For this review, take the finished solid that the model builds, in its own axes (mm). Face numbers are marked on the shaded views. A direction names the side the tool comes from. Give positions to 0.01 mm unless a question says otherwise; leave off trailing zeros. Write each loop counter-clockwise with the first axis right and the second up, starting at its lowest first coordinate (ties: lowest second). Pieces come first, ordered by that corner, then holes. Notation, with made-up numbers: M -16.5,-37.75 L 36.5,-37.75 A26 ccw 36.5,-15.75 Z; hole C 30,9.25 d7. An arc over 180 degrees is marked long. One line per item, written item: value. Start each with the question number.
Item 1: Tool access review of the marked faces 4 and 5: name each direction out of +Z, -Z, +X, -X, +Y, -Y from which nothing blocks a thin tool from reaching the whole face with its end or side.
Item 2: Consider section C-C, the plane z = 35.5. Write out the cut boundary in (x, y).
Item 3: Clearance check with flat-ended pins moving along their axes: pin 1 Ø0.6 at (y, z) = (3.5, 15.5) entering from +X; pin 2 Ø2 at (x, y) = (1, 2.5) entering from -Z; pin 3 Ø1.9 at (y, z) = (-3.5, 4.5) entering from -X; pin 4 Ø0.9 at (x, z) = (0, 2.75) entering from +Y. State where each tip first meets the part, or that it passes through.
Item 4: Consider section B-B, the plane z = 4.5. Write out the cut boundary in (x, y).
Item 5: To check wall thickness, follow probe 1 along X at (y, z) = (-4.95, 2.75); probe 2 along Z at (x, y) = (0, -4.35); probe 3 along Y at (x, z) = (2.25, 35.5). State the ranges of each line that lie inside material, in increasing order.
Item 6: Mouldability with a two-part tool opening along Y and no side actions: class the marked faces 1, 2 and 3 as released by +Y, released by -Y, zero draft, split by the parting line, or undercut.
Item 7: Consider section A-A, the plane x = 0. Write out the cut boundary in (y, z).
Item 8: Consider section D-D, the plane y = -4.25. Write out the cut boundary in (x, z), and give its area (3 significant figures).
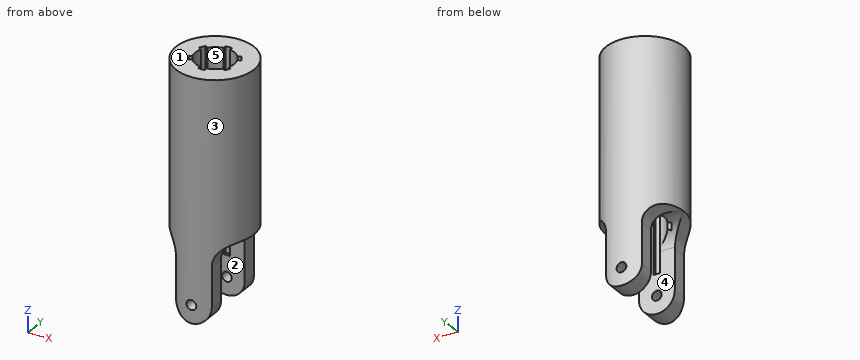
```python
from build123d import *

# Parameters (mm, degrees)
SKETCH_1_R          = 6
SKETCH_1_R_2        = 2.5
EXTRUDE_1_DEPTH     = 37
SKETCH_2_OUTSIDE_W  = 22.142
SKETCH_2_OUTSIDE_H  = 47.142
SKETCH_2_OUTSIDE_R  = 0.75
CUT_EXTRUDE_1_DEPTH = 9.5
CUT_EXTRUDE_2_DEPTH = 9.5
CUT_EXTRUDE_3_DEPTH = 31


with BuildPart() as part:
    # 草图1 → 凸台-拉伸1 (new body)
    with BuildSketch(Plane.XY):
        Circle(SKETCH_1_R)
        Circle(SKETCH_1_R_2, mode=Mode.SUBTRACT)
    extrude(amount=EXTRUDE_1_DEPTH)

    # 草图2 outside → 切除-拉伸1 (cut, symmetric)
    with BuildSketch(Plane(origin=(0, 0, 0), x_dir=(1, 0, 0), z_dir=(0, 1, 0))):
        with Locations((0, -18.5)):
            Rectangle(SKETCH_2_OUTSIDE_W, SKETCH_2_OUTSIDE_H)
        with BuildLine():
            Line((-2.75, -2.75), (-2.75, -9))
            ThreePointArc((-2.75, -9), (-3.701902961, -11.298097039), (-6, -12.25))
            Line((-6, -12.25), (-6, -37))
            Line((-6, -37), (6, -37))
            Line((6, -37), (6, -12.25))
            ThreePointArc((6, -12.25), (3.701902961, -11.298097039), (2.75, -9))
            Line((2.75, -9), (2.75, -2.75))
            ThreePointArc((2.75, -2.75), (0, 0), (-2.75, -2.75))
        make_face(mode=Mode.SUBTRACT)
        with Locations((0, -2.75)):
            Circle(SKETCH_2_OUTSIDE_R)
    extrude(amount=CUT_EXTRUDE_1_DEPTH, both=True, mode=Mode.SUBTRACT)

    # 草图3 → 切除-拉伸2 (cut, symmetric)
    with BuildSketch(Plane(origin=(0, 0, 0), x_dir=(0, 0, -1), z_dir=(1, 0, 0))):
        with BuildLine():
            Line((-9.250000001, 3), (0.966464558, 3))
            Line((0.966464558, 3), (0.966464558, -3))
            Line((0.966464558, -3), (-9.250000001, -3))
            ThreePointArc((-9.250000001, -3), (-12.250000001, 0), (-9.250000001, 3))
        make_face()
    extrude(amount=CUT_EXTRUDE_2_DEPTH, both=True, mode=Mode.SUBTRACT)

    # 草图4 → 切除-拉伸3 (cut)
    with BuildSketch(Plane.XY.offset(37)):
        with BuildLine():
            Line((-0.5, 3.464101615), (-0.5, 2.958039892))
            ThreePointArc((-0.5, 2.958039892), (-1.5, 2.598076211), (-2.311737691, 1.912032648))
            Line((-2.311737691, 1.912032648), (-2.75, 2.165063509))
            ThreePointArc((-2.75, 2.165063509), (-3.031088913, 1.75), (-3.25, 1.299038106))
            Line((-3.25, 1.299038106), (-2.811737691, 1.046007244))
            ThreePointArc((-2.811737691, 1.046007244), (-3, 0), (-2.811737691, -1.046007244))
            Line((-2.811737691, -1.046007244), (-3.25, -1.299038106))
            ThreePointArc((-3.25, -1.299038106), (-3.031088913, -1.75), (-2.75, -2.165063509))
            Line((-2.75, -2.165063509), (-2.311737691, -1.912032648))
            ThreePointArc((-2.311737691, -1.912032648), (-1.5, -2.598076211), (-0.5, -2.958039892))
            Line((-0.5, -2.958039892), (-0.5, -3.464101615))
            ThreePointArc((-0.5, -3.464101615), (0, -3.5), (0.5, -3.464101615))
            Line((0.5, -3.464101615), (0.5, -2.958039892))
            ThreePointArc((0.5, -2.958039892), (1.5, -2.598076211), (2.311737691, -1.912032648))
            Line((2.311737691, -1.912032648), (2.75, -2.165063509))
            ThreePointArc((2.75, -2.165063509), (3.031088913, -1.75), (3.25, -1.299038106))
            Line((3.25, -1.299038106), (2.811737691, -1.046007244))
            ThreePointArc((2.811737691, -1.046007244), (3, 0), (2.811737691, 1.046007244))
            Line((2.811737691, 1.046007244), (3.25, 1.299038106))
            ThreePointArc((3.25, 1.299038106), (3.031088913, 1.75), (2.75, 2.165063509))
            Line((2.75, 2.165063509), (2.311737691, 1.912032648))
            ThreePointArc((2.311737691, 1.912032648), (1.5, 2.598076211), (0.5, 2.958039892))
            Line((0.5, 2.958039892), (0.5, 3.464101615))
            ThreePointArc((0.5, 3.464101615), (0, 3.5), (-0.5, 3.464101615))
        make_face()
    extrude(amount=-CUT_EXTRUDE_3_DEPTH, mode=Mode.SUBTRACT)


solid = part.part
```
Model answer:
1. face 4: -Z, +X, -X
1. face 5: +Z, -Z
2. outline: C 0,0 d12; hole M -3.25,-1.3 A3.5 ccw -2.75,-2.17 L -2.31,-1.91 A3 ccw -0.5,-2.96 L -0.5,-3.46 A3.5 ccw 0.5,-3.46 L 0.5,-2.96 A3 ccw 2.31,-1.91 L 2.75,-2.17 A3.5 ccw 3.25,-1.3 L 2.81,-1.05 A3 ccw 2.81,1.05 L 3.25,1.3 A3.5 ccw 2.75,2.17 L 2.31,1.91 A3 ccw 0.5,2.96 L 0.5,3.46 A3.5 ccw -0.5,3.46 L -0.5,2.96 A3 ccw -2.31,1.91 L -2.75,2.17 A3.5 ccw -3.25,1.3 L -2.81,1.05 A3 ccw -2.81,-1.05 Z
3. pin 1: stops at x = 5.08
3. pin 2: stops at z = 0
3. pin 3: stops at x = -2.75
3. pin 4: passes through
4. outline: M -2.75,-5.33 A6 ccw 2.75,-5.33 L 2.75,-3 L -2.75,-3 Z; M -2.75,3 L 2.75,3 L 2.75,5.33 A6 ccw -2.75,5.33 Z
5. probe 1: x = -2.75 to -0.75, 0.75 to 2.75
5. probe 2: z = 0 to 2, 3.5 to 37
5. probe 3: y = -5.56 to -1.98, 1.98 to 5.56
6. face 1: zero draft
6. face 2: undercut
6. face 3: split by the parting line
7. outline: M -6,0 L -3,0 L -3,2 L -6,2 Z; M -6,3.5 L -3,3.5 L -3,6 L -3.5,6 L -3.5,37 L -6,37 Z; M 3,0 L 6,0 L 6,2 L 3,2 Z; M 3,3.5 L 6,3.5 L 6,37 L 3.5,37 L 3.5,6 L 3,6 Z
8. outline: M -4.24,11.73 A3.25 cw -2.75,9 L -2.75,2.75 A2.75 ccw 2.75,2.75 L 2.75,9 A3.25 cw 4.24,11.73 L 4.24,37 L -4.24,37 Z; hole C 0,2.75 d1.5
8. area: 276 mm2
